Design review of the part shown in the three views and the two pictorial views. Dimensions are in mm from the part's minimum x, y and z. Round coordinates to 2 decimals unless told otherwise and drop trailing zeros. Write each loop counter-clockwise with the first axis right and the second up, starting at its lowest first coordinate (ties: lowest second). Pieces come first, ordered by that corner, then holes. Notation, with made-up numbers: (47, 71) -> (76, 71) arc R16 ccw to (76, 85) -> close; hole circle Ø1 at (-31, -1). An arc over 180 degrees is marked (long way). One line per question, with ' | ' between items. Start each with the question number.
1) Insertion check: pin 1 Ø1.4 at (x, z) = (4.175, 55.825) entering from -Y; pin 2 Ø8 at (x, z) = (63, 12) entering from -Y. Each pin has a flat end and moves straight along its axis. Give the tip position at first contact, or say it passes through.
2) Consider section C-C (z = 43.5). Give the boundary of the cut face in (x, y).
3) Consider section D-D (y = 0.6). Count the separate pieces of the cut face and the enclosed holes in it.
4) Consider section B-B (x = 28). Give the boundary of the cut face in (y, z).
5) For probe 1 along X at (y, z) = (1.5, 44); probe 2 along X at (y, z) = (0.25, 16); probe 3 along Z at (x, y) = (31, 1.1), list the stretches that pass through material, from the lowest coordinate up.
6) Consider section A-A (z = 26.5). Give the boundary of the cut face in (x, y).
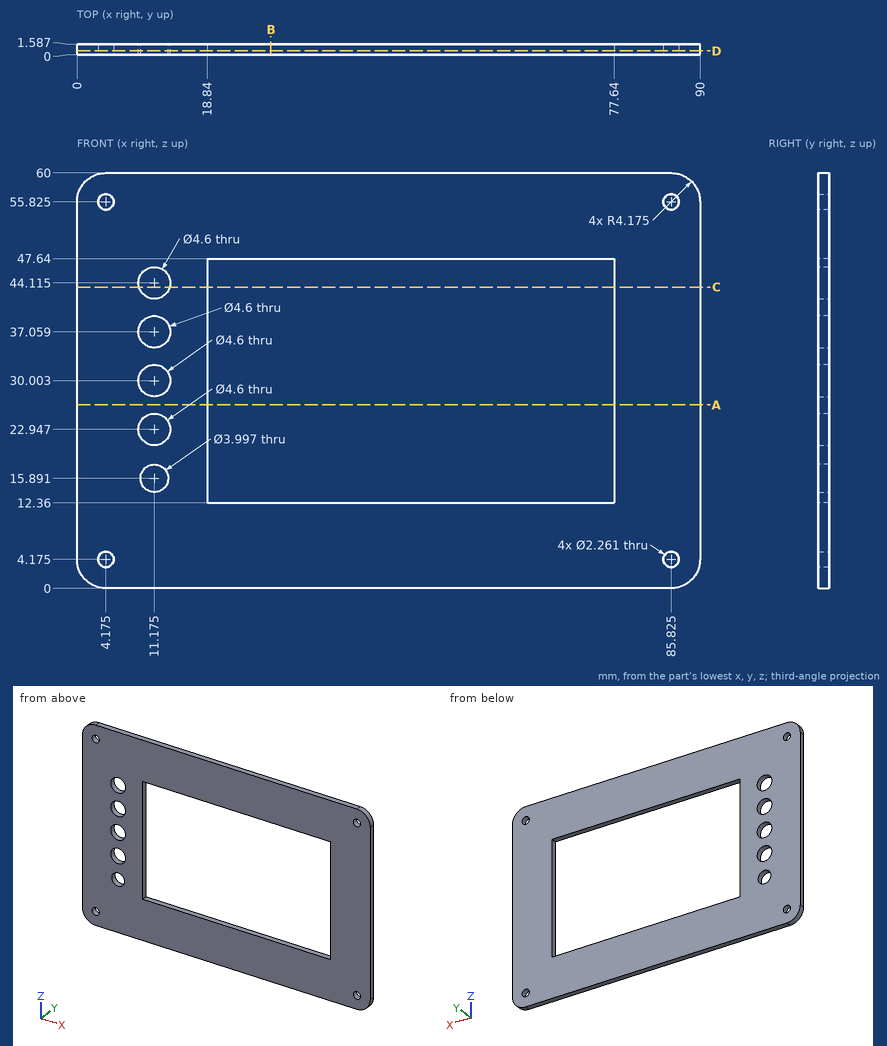
From the geometry:
1) pin 1: passes through | pin 2: stops at y = 0
2) outline: (0, 0) -> (8.96, 0) -> (8.96, 1.59) -> (0, 1.59) -> close; (13.39, 0) -> (18.84, 0) -> (18.84, 1.59) -> (13.39, 1.59) -> close; (77.64, 0) -> (90, 0) -> (90, 1.59) -> (77.64, 1.59) -> close
3) separate pieces: 1 | enclosed holes: 10
4) outline: (0, 0) -> (1.59, 0) -> (1.59, 12.36) -> (0, 12.36) -> close; (0, 47.64) -> (1.59, 47.64) -> (1.59, 60) -> (0, 60) -> close
5) probe 1: x = 0 to 8.88, 13.47 to 18.84, 77.64 to 90 | probe 2: x = 0 to 9.18, 13.17 to 18.84, 77.64 to 90 | probe 3: z = 0 to 12.36, 47.64 to 60
6) outline: (0, 0) -> (18.84, 0) -> (18.84, 1.59) -> (0, 1.59) -> close; (77.64, 0) -> (90, 0) -> (90, 1.59) -> (77.64, 1.59) -> close
